from build123d import *

# Parameters (mm, degrees)
BOSS_EXTRUDE1_DEPTH                                 = 6
CSK_FOR_M5_COUNTERSUNK_FLAT_HEAD_SCREW1_D           = 5.3
CSK_FOR_M5_COUNTERSUNK_FLAT_HEAD_SCREW1_CSINK_D     = 10.4
CSK_FOR_M5_COUNTERSUNK_FLAT_HEAD_SCREW1_CSINK_ANGLE = 90
F_2_6_2_6_DIAMETER_HOLE1_D                          = 2.6
FILLET1_R                                           = 10
FILLET2_R                                           = 1


with BuildPart() as part:
    # Sketch1 → Boss-Extrude1 (new body)
    with BuildSketch(Plane.XY):
        with BuildLine():
            Line((-15, -10), (-15, 0))
            Line((-15, 0), (-52, 0))
            Line((-52, 0), (-52, -500))
            Line((-52, -500), (-15, -500))
            Line((-15, -500), (-15, -490))
            ThreePointArc((-15, -490), (-13.535533906, -486.464466094), (-10, -485))
            Line((-10, -485), (10, -485))
            ThreePointArc((10, -485), (13.535533906, -486.464466094), (15, -490))
            Line((15, -490), (15, -500))
            Line((15, -500), (52, -500))
            Line((52, -500), (52, 0))
            Line((52, 0), (15, 0))
            Line((15, 0), (15, -10))
            ThreePointArc((15, -10), (13.535533906, -13.535533906), (10, -15))
            Line((10, -15), (-10, -15))
            ThreePointArc((-10, -15), (-13.535533906, -13.535533906), (-15, -10))
        make_face()
        with BuildLine():
            ThreePointArc((-15, -340), (-13.535533906, -336.464466094), (-10, -335))
            Line((-10, -335), (10, -335))
            ThreePointArc((10, -335), (13.535533906, -336.464466094), (15, -340))
            Line((15, -340), (15, -460))
            ThreePointArc((15, -460), (13.535533906, -463.535533906), (10, -465))
            Line((10, -465), (-10, -465))
            ThreePointArc((-10, -465), (-13.535533906, -463.535533906), (-15, -460))
            Line((-15, -460), (-15, -340))
        make_face(mode=Mode.SUBTRACT)
        with BuildLine():
            ThreePointArc((-15, -190), (-13.535533906, -186.464466094), (-10, -185))
            Line((-10, -185), (10, -185))
            ThreePointArc((10, -185), (13.535533906, -186.464466094), (15, -190))
            Line((15, -190), (15, -310))
            ThreePointArc((15, -310), (13.535533906, -313.535533906), (10, -315))
            Line((10, -315), (-10, -315))
            ThreePointArc((-10, -315), (-13.535533906, -313.535533906), (-15, -310))
            Line((-15, -310), (-15, -190))
        make_face(mode=Mode.SUBTRACT)
        with BuildLine():
            ThreePointArc((-15, -40), (-13.535533906, -36.464466094), (-10, -35))
            Line((-10, -35), (10, -35))
            ThreePointArc((10, -35), (13.535533906, -36.464466094), (15, -40))
            Line((15, -40), (15, -160))
            ThreePointArc((15, -160), (13.535533906, -163.535533906), (10, -165))
            Line((10, -165), (-10, -165))
            ThreePointArc((-10, -165), (-13.535533906, -163.535533906), (-15, -160))
            Line((-15, -160), (-15, -40))
        make_face(mode=Mode.SUBTRACT)
    extrude(amount=BOSS_EXTRUDE1_DEPTH)

    # CSK for M5 Countersunk Flat Head Screw1 (through all)
    with Locations(Plane.XY.offset(6)):
        with Locations((30, -480), (-30, -20), (30, -20), (-30, -90.666666667), (30, -90.666666667), (-30, -170.333333333), (30, -170.333333333), (30, -250), (-30, -250), (-30, -320.666666667), (30, -320.666666667), (-30, -400.333333333), (30, -400.333333333), (-30, -480)):
            CounterSinkHole(CSK_FOR_M5_COUNTERSUNK_FLAT_HEAD_SCREW1_D / 2, CSK_FOR_M5_COUNTERSUNK_FLAT_HEAD_SCREW1_CSINK_D / 2, counter_sink_angle=CSK_FOR_M5_COUNTERSUNK_FLAT_HEAD_SCREW1_CSINK_ANGLE)

    # Ø2.6 (2.6) Diameter Hole1 (through all)
    with Locations(Plane.XY.offset(6)):
        with Locations((-46, -510), (-46, -10), (46, -10), (46, -35), (46, -60), (46, -85), (46, -110), (46, -135), (46, -160), (46, -185), (46, -210), (46, -235), (46, -260), (46, -285), (46, -310), (46, -335), (46, -360), (46, -385), (46, -410), (46, -435), (46, -460), (46, -485), (46, -510), (-46, -35), (-46, -60), (-46, -85), (-46, -110), (-46, -135), (-46, -160), (-46, -185), (-46, -210), (-46, -235), (-46, -260), (-46, -285), (-46, -310), (-46, -335), (-46, -360), (-46, -385), (-46, -410), (-46, -435), (-46, -460), (-46, -485)):
            Hole(F_2_6_2_6_DIAMETER_HOLE1_D / 2)

    # Fillet1
    fillet1_edges = [part.edges().sort_by_distance(p)[0] for p in [
        (15, 0, 3),
        (-15, 0, 3),
        (15, -500, 3),
        (-15, -500, 3),
    ]]
    fillet(fillet1_edges, radius=FILLET1_R - 0.0001)  # a hair under: the kernel refuses the full size

    # Fillet2
    fillet2_edges = [part.edges().sort_by_distance(p)[0] for p in [
        (-52, -500, 3),
        (-52, 0, 3),
        (52, 0, 3),
        (52, -500, 3),
    ]]
    fillet(fillet2_edges, radius=FILLET2_R)


solid = part.part
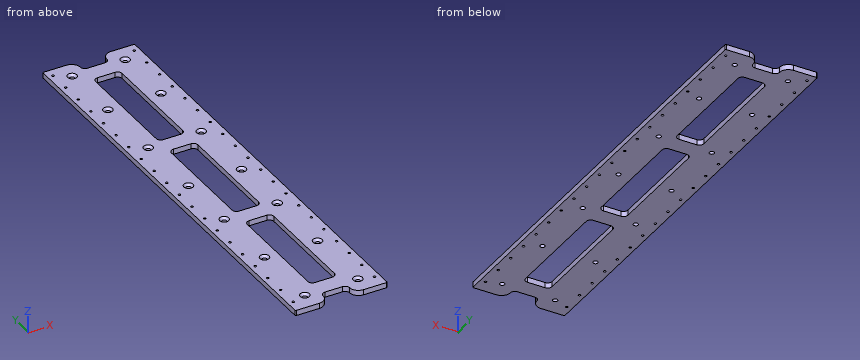
The listing builds one solid part. Answer for the finished solid, in the listing's coordinates (mm). Round coordinates to 2 decimals unless told otherwise and drop trailing zeros. Loops run counter-clockwise (first coordinate to the right, second up) from the corner with the lowest first, then second, coordinate; pieces in that order, holes last. Notation, with made-up numbers: M -33.75,47.5 L 10.25,47.5 A27 cw 10.25,81.5 Z; hole C 41,-8.75 d7. An arc over 180 degrees is marked long. Return JSON: item names as keys, results as strings.
Q1. Find section A-A, the plane y = -202. Determine the outline of the cut face in (x, z), plus the area to 3 significant figures.
Results list:
{"outline": "M -52,0 L -15,0 L -15,6 L -52,6 Z; M 15,0 L 52,0 L 52,6 L 15,6 Z", "area": "444 mm2"}
Q2. Each of these flat-tipped pins is pushed along its axis until it touches: pin 1 Ø3 at (x, z) = (-1.5, 4) entering from -Y; pin 2 Ø8.5 at (x, y) = (-30, -20) entering from +Z. Where does it stop, or does it pass through?
Results list:
{"pin 1": "stops at y = -485", "pin 2": "stops at z = 5.05"}
Q3. Find section B-B, the plane z = 4.75. State how many separate pieces and enclosed holes the cut face has, plus the area to 3 significant figures.
Results list:
{"separate pieces": "1", "enclosed holes": "57", "area": "38,500 mm2"}
Q4. Find the intervals of material crossed by line 1 along Y through (x, z) = (7.5, 4.75); line 2 along X through (y, z) = (-310, 2.6); line 3 along X through (y, z) = (-215, 3.4), in increasing order. Write a range as from..to.
Results list:
{"line 1": "y = -485..-465, -335..-315, -185..-165, -35..-15", "line 2": "x = -52..-47.3, -44.7..-15, 15..44.7, 47.3..52", "line 3": "x = -52..-15, 15..52"}
